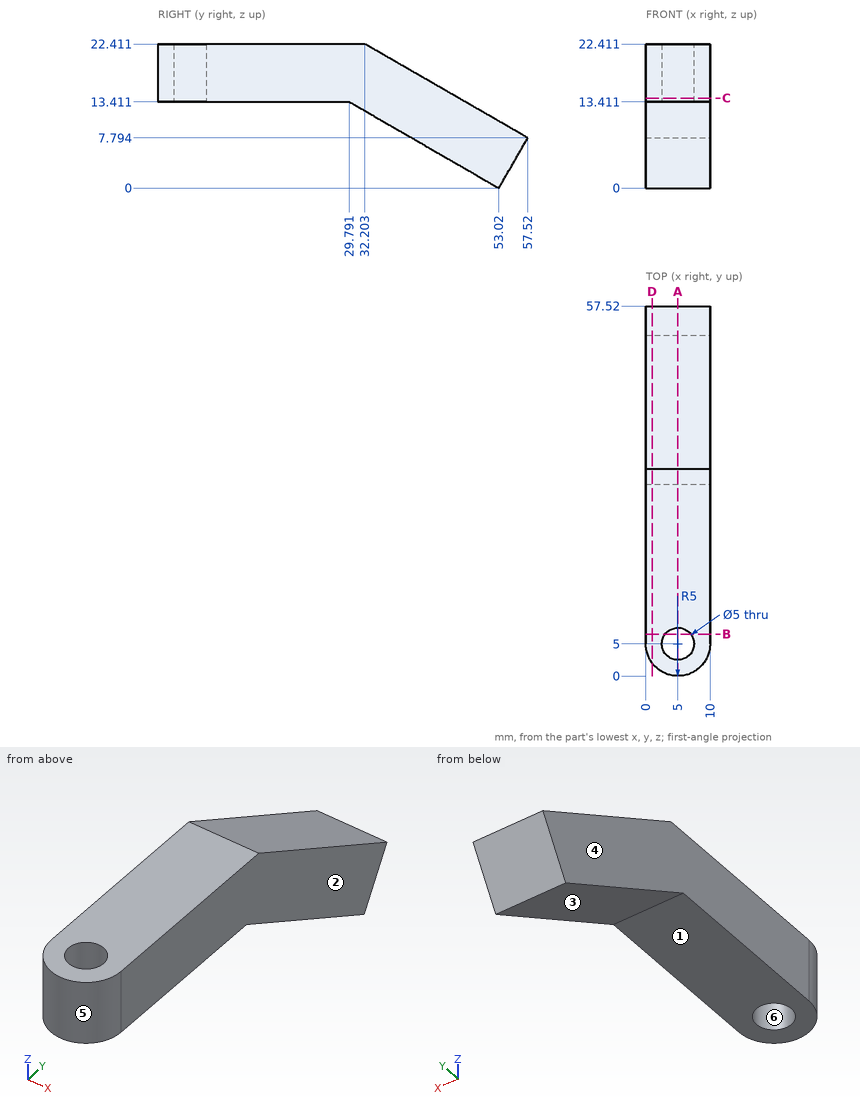
Design review of the part shown in the three views and the two pictorial views. Dimensions are in mm from the part's minimum x, y and z. A direction names the side the tool comes from. Round coordinates to 2 decimals unless told otherwise and drop trailing zeros. Loops run counter-clockwise (first coordinate to the right, second up) from the corner with the lowest first, then second, coordinate; pieces in that order, holes last.
Q1. Add section A-A on x = 5. Write out the cut boundary in (y, z) (1 decimal).
Result sheet:
outline: (0, 13.4) - (2.5, 13.4) - (2.5, 22.4) - (0, 22.4) - close; (7.5, 13.4) - (29.8, 13.4) - (53, 0) - (57.5, 7.8) - (32.2, 22.4) - (7.5, 22.4) - close
Q2. Mouldability with a two-part tool opening along X and no side actions: class the marked faces 3, 4, 5 and 6 as +X half, -X half, draft (parallel to the pull), parting line (faces both ways), or undercut.
Result sheet:
face 3: draft
face 4: -X half
face 5: parting line
face 6: undercut
Q3. Add section C-C on z = 14. Write out the cut boundary in (x, y), plus the area to 3 significant figures.
Result sheet:
outline: (0, 5) arc R5 ccw to (10, 5) - (10, 46.77) - (0, 46.77) - close; hole circle Ø5 at (5, 5)
area: 437 mm2
Q4. Add section D-D on x = 1. Write out the cut boundary in (y, z) (1 decimal), plus the area to 3 significant figures.
Result sheet:
outline: (2, 13.4) - (29.8, 13.4) - (53, 0) - (57.5, 7.8) - (32.2, 22.4) - (2, 22.4) - close
area: 513 mm2
Q5. Add section B-B on y = 6.5. Write out the cut boundary in (x, z), plus the area to 3 significant figures.
Result sheet:
outline: (0, 13.41) - (3, 13.41) - (3, 22.41) - (0, 22.41) - close; (7, 13.41) - (10, 13.41) - (10, 22.41) - (7, 22.41) - close
area: 54.0 mm2
Q6. Machinability: for the marked faces 1 and 2, which of the approach directions +Z, -Z, +X, -X, +Y, -Y give a long, thin tool a straight path to every point of the face, cutting with its end or side? Answer none if there is none.
Result sheet:
face 1: -Z, +X, -X, -Y
face 2: +Z, -Z, +X, +Y, -Y
Q7. Insertion check: pin 1 Ø1 at (y, z) = (51, 11) entering from -X; pin 2 Ø3 at (x, y) = (6, 13.5) entering from -Z. Each pin has a flat end and moves straight along its axis. Give the tip position at first contact, or say it passes through.
Result sheet:
pin 1: stops at x = 0
pin 2: stops at z = 13.41
Q8. To check wall thickness, follow line 1 along X through (y, z) = (5, 20.25); line 2 along Z through (x, y) = (2, 12.5); line 3 along Y through (x, z) = (5.75, 17) (1 decimal). State the ranges of each line that lie inside material, in increasing order.
Result sheet:
line 1: x = 0 to 2.5, 7.5 to 10
line 2: z = 13.41 to 22.41
line 3: y = 0.1 to 2.6, 7.4 to 41.6
